Work out the finished part from the listing and answer in its coordinate system (mm). Face numbers are marked on the shaded views. A direction names the side the tool comes from. Coordinates: 2 decimals unless noted, no trailing zeros. Loops run counter-clockwise (first coordinate to the right, second up) from the corner with the lowest first, then second, coordinate; pieces in that order, holes last. Notation, with made-up numbers: (-4.5, 20.5) - (39.5, 20.5) arc R26 cw to (39.5, 36.5) - close; hole circle Ø3 at (86, 71). An arc over 180 degrees is marked (long way). Write each question's results on one line, items separated by ' | '. Start each with the question number.
1. Which of the six approach directions +Z, -Z, +X, -X, +Y, -Y give full straight-line access (tool end or side, diameter ignored) to the marked faces 5, 6 and 7?
2. A cutting plane is placed at B-B on y = -1.5. Determine the outline of the cut face in (x, z), then the cut area to 3 significant figures.
3. Find the intervals of material crossed by line 1 along Z through (x, y) = (5, -10.25); line 2 along Y through (x, z) = (8.5, -12); line 3 along X through (y, z) = (-3.75, -24), in increasing order. Write a range as [from, to].
4. Each of these flat-tipped pins is pushed along its axis until it touches: P1, Ø6, axis at x = 5, z = -22, coming from the -Y side; P2, Ø8, axis at y = -17.5, z = -7, coming from the +X side; P3, Ø3.5, axis at x = 15, z = -8.5, coming from the +Y side. Where does it stop, or does it pass through?
5. Determine the mould class of the marked faces 1, 2, 3 and 4 for opening direction Z: released by +Z, released by -Z, zero draft, split by the parting line, or undercut.
6. A cutting plane is placed at A-A on x = 17. Determine the outline of the cut face in (y, z), then the cut area to 3 significant figures.
7. A cutting plane is placed at D-D on x = 5. Determine the outline of the cut face in (y, z), then the cut area to 3 significant figures.
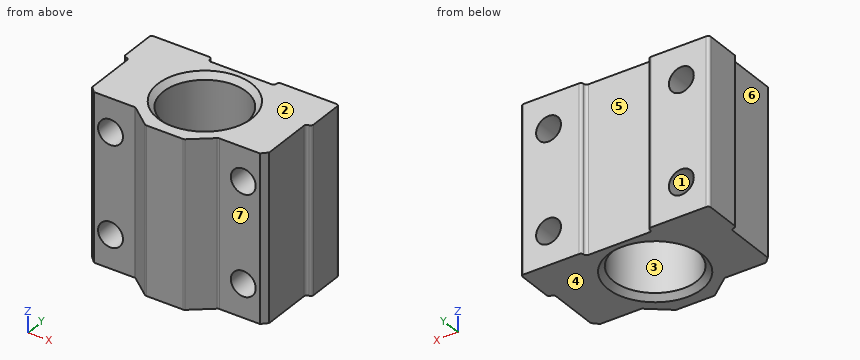
from build123d import *

# Parameters (mm, degrees)
ESTRUSIONE_ESTRUSIONE1_DEPTH = 30
SCHIZZO3_R                   = 7.5
TAGLIO_ESTRUSIONE2_DEPTH     = 50.969990995
SMUSSO1_SIZE                 = 1
RACCORDO1_R                  = 0.5
FORO_PER_VITE_M4_1_D         = 4.5


with BuildPart() as part:
    # Schizzo2 → Estrusione-Estrusione1 (new body)
    with BuildSketch(Plane.XY):
        Polygon((0, 0), (11, 0), (11, -1), (23, -1), (23, 0), (34, 0), (34, -7.2), (33, -7.2), (33, -17.8), (24.5, -17.8), (20.5, -21), (13.5, -21), (9.5, -17.8), (1, -17.8), (1, -7.2), (0, -7.2), align=None)
    extrude(amount=-ESTRUSIONE_ESTRUSIONE1_DEPTH)

    # Schizzo3 → Taglio-Estrusione2 (cut, through all)
    with BuildSketch(Plane.XY):
        with Locations((17, -10.5)):
            Circle(SCHIZZO3_R)
    extrude(amount=-TAGLIO_ESTRUSIONE2_DEPTH, mode=Mode.SUBTRACT)

    # Smusso1
    smusso1_edges = [part.edges().sort_by_distance(p)[0] for p in [
        (33, -17.8, -15),
        (1, -17.8, -15),
        (9.5, -10.5, -30),
        (9.5, -10.5, 0),
    ]]
    chamfer(smusso1_edges, length=SMUSSO1_SIZE)

    # Raccordo1
    raccordo1_edges = [part.edges().sort_by_distance(p)[0] for p in [
        (9.5, -17.8, -15),
        (24.5, -17.8, -15),
        (20.5, -21, -15),
        (13.5, -21, -15),
        (1, -7.2, -15),
        (0, -7.2, -15),
        (0, 0, -15),
        (23, -1, -15),
        (11, -1, -15),
        (11, 0, -15),
        (23, 0, -15),
        (34, 0, -15),
        (34, -7.2, -15),
        (33, -7.2, -15),
    ]]
    fillet(raccordo1_edges, radius=RACCORDO1_R - 0.0001)  # a hair under: the kernel refuses the full size

    # Foro per Vite M4-1 (through all)
    with Locations(Plane(origin=(0, 0, 0), x_dir=(1, 0, 0), z_dir=(0, 1, 0))):
        with Locations((29, 24), (29, 6), (5, 6), (5, 24)):
            Hole(FORO_PER_VITE_M4_1_D / 2)


solid = part.part
Values:
1) face 5: +Z, -Z, +Y | face 6: +Z, -Z, -X, -Y | face 7: +Z, -Z, +X, -Y
2) outline: (0, -30) - (34, -30) - (34, 0) - (0, 0) - close; hole circle Ø4.5 at (5, -24); hole circle Ø4.5 at (5, -6); hole circle Ø4.5 at (29, -24); hole circle Ø4.5 at (29, -6) | area: 956 mm^2
3) line 1: [-30, -26.25], [-21.75, -8.25], [-3.75, 0] | line 2: [-17.8, 0] | line 3: [0, 2.75], [7.25, 13.73], [20.27, 26.75], [31.25, 34]
4) P1: y = -17.8 | P2: x = 33 | P3: y = -1
5) face 1: undercut | face 2: released by +Z | face 3: zero draft | face 4: released by -Z
6) outline: (-21, -30) - (-19, -30) - (-18, -29) - (-18, -1) - (-19, 0) - (-21, 0) - close; (-3, -29) - (-2, -30) - (-1, -30) - (-1, 0) - (-2, 0) - (-3, -1) - close | area: 148 mm^2
7) outline: (-17.8, -30) - (0, -30) - (0, -26.25) - (-17.8, -26.25) - close; (-17.8, -21.75) - (0, -21.75) - (0, -8.25) - (-17.8, -8.25) - close; (-17.8, -3.75) - (0, -3.75) - (0, 0) - (-17.8, 0) - close | area: 374 mm^2
